from build123d import *

# Parameters (mm, degrees)
SKETCH1_W                  = 88.9
SKETCH1_H                  = 25.4
BOSS_EXTRUDE1_DEPTH        = 3.175
SKETCH2_R                  = 4.7625
SKETCH2_R_2                = 2.0955
CUT_EXTRUDE1_DEPTH         = 3.175
CONVERT_SOLID1_OUTLINE_W   = 88.9
CONVERT_SOLID1_OUTLINE_H   = 25.4
CONVERT_SOLID1_OUTLINE_R   = 2.0955
CONVERT_SOLID1_OUTLINE_R_2 = 4.7625
CONVERT_SOLID1_DEPTH       = 0.635


# Read off the part's stored shape, not the designer's step: Convert-Solid1
with BuildPart() as part:
    # Sketch1 → Boss-Extrude1 (new body)
    with BuildSketch(Plane(origin=(0, 0, 0), x_dir=(1, 0, 0), z_dir=(0, 1, 0))):
        with Locations((44.45, 12.7)):
            Rectangle(SKETCH1_W, SKETCH1_H)
    extrude(amount=BOSS_EXTRUDE1_DEPTH)

    # Sketch2 → Cut-Extrude1 (cut)
    with BuildSketch(Plane(origin=(0, 3.175, 0), x_dir=(1, 0, 0), z_dir=(0, 1, 0))):
        with Locations(Location((76.2, 12.7, 0), (0, 0, 270))):
            Circle(SKETCH2_R)
        with Locations(Location((5.715, 19.05, 0), (0, 0, 270))):
            Circle(SKETCH2_R_2)
        with Locations(Location((17.145, 6.35, 0), (0, 0, 270))):
            Circle(SKETCH2_R_2)
    extrude(amount=-CUT_EXTRUDE1_DEPTH, mode=Mode.SUBTRACT)

    # Convert-Solid1 outline → Convert-Solid1 (cut)
    with BuildSketch(Plane(origin=(0, 0, 0), x_dir=(1, 0, 0), z_dir=(0, 1, 0))):
        with Locations((44.45, 12.7)):
            Rectangle(CONVERT_SOLID1_OUTLINE_W, CONVERT_SOLID1_OUTLINE_H)
        with Locations((17.145, 6.35)):
            Circle(CONVERT_SOLID1_OUTLINE_R, mode=Mode.SUBTRACT)
        with Locations((76.2, 12.7)):
            Circle(CONVERT_SOLID1_OUTLINE_R_2, mode=Mode.SUBTRACT)
        with Locations((5.715, 19.05)):
            Circle(CONVERT_SOLID1_OUTLINE_R, mode=Mode.SUBTRACT)
    extrude(amount=CONVERT_SOLID1_DEPTH, mode=Mode.SUBTRACT)


solid = part.part
The listing builds one solid part. Answer for the finished solid, in the listing's coordinates (mm). Round coordinates to 2 decimals unless told otherwise and drop trailing zeros. Write each loop counter-clockwise with the first axis right and the second up, starting at its lowest first coordinate (ties: lowest second). Pieces come first, ordered by that corner, then holes. Notation, with made-up numbers: (-19.75, 21.5) - (4.25, 21.5) arc R22 cw to (4.25, 48.5) - close; hole circle Ø1 at (34.25, 21.25). An arc over 180 degrees is marked (long way). Use one line per item in the form item = value. Start each with the question number.
Item 1: A cutting plane is placed at A-A (z = -12.7). Write down the section's boundary in (x, y) (1 decimal), plus the area to 3 significant figures.
Item 2: A flat-ended cylindrical pin translates along its axis: pin 1 Ø5 at (x, z) = (17.145, -6.35) entering from +Y (3 decimals). Find the tip coordinate at first contact, or state that the pin passes through.
Item 3: A cutting plane is placed at C-C (y = 1.6). Give the number of separate pieces and of enclosed holes in the cut face, plus the area to 3 significant figures.
Item 4: A cutting plane is placed at B-B (x = 76.2). Write down the section's boundary in (y, z) (1 decimal), plus the area to 3 significant figures.
Item 5: Determine the mould class of faces 1 (the flat face through (88.9, 2, -13)), 2 (the cylindrical face through (76.409, 1.923, -17.458)), 3 (the flat face through (44, 0.635, -13)) for opening direction X: +X half, -X half, draft (parallel to the pull), parting line (faces both ways), or undercut.
Item 6: Find the intervals of material crossed by line 1 (X direction, y = 1.25, z = -19.05); line 2 (Z direction, x = 76.2, y = 2.4); line 3 (X direction, y = 1.95, z = -14.5), in increasing order. Write a range as [from, to].
The answers:
q1.outline = (0, 0.6) - (71.4, 0.6) - (71.4, 3.2) - (0, 3.2) - close; (81, 0.6) - (88.9, 0.6) - (88.9, 3.2) - (81, 3.2) - close
q1.area = 202 mm^2
q2.pin_1 = 3.175
q3.separate_pieces = 1
q3.enclosed_holes = 3
q3.area = 2,160 mm^2
q4.outline = (0.6, -25.4) - (3.2, -25.4) - (3.2, -17.5) - (0.6, -17.5) - close; (0.6, -7.9) - (3.2, -7.9) - (3.2, 0) - (0.6, 0) - close
q4.area = 40.3 mm^2
q5.face_1 = +X half
q5.face_2 = undercut
q5.face_3 = draft
q6.line_1 = [0, 3.62], [7.81, 88.9]
q6.line_2 = [-25.4, -17.46], [-7.94, 0]
q6.line_3 = [0, 71.79], [80.61, 88.9]
